Can you work these out from the model? Positions are in its coordinate system, mm. A direction names the side the tool comes from. Round coordinates to 2 decimals unless told otherwise and drop trailing zeros. Order: outer loops, then holes, each group sorted by start corner. A loop starts at its lowest first (then second) coordinate and runs counter-clockwise, first axis right, second up. Notation, with made-up numbers: (10.25, -14.75) - (59.25, -14.75) arc R32 ccw to (59.25, 16.25) - close; hole circle Ø9 at (54, 76.5). An arc over 180 degrees is marked (long way). Write item = value, one per line.
Autodesk Inventor part; units mm, degrees
ref_plane "YZ Plane" through (0, 0, 0) normal (1, 0, 0) x (0, 1, 0)
ref_plane "XZ Plane" through (0, 0, 0) normal (0, 1, 0) x (-1, 0, 0)
ref_plane "XY Plane" through (0, 0, 0) normal (0, 0, 1) x (1, 0, 0)
sketch "Sketch1" plane through (0, 0, 0) normal (0, 0, 1) x (1, 0, 0)
  circle A0 centre (0, 0) radius 107.6 construction
  arc A1 (43.4971, -89.6) -> (-43.4971, -89.6) centre (0, 0) ccw construction
  line L0 (43.4971, -89.6) -> (-43.4971, -89.6) construction
  arc A2 (-96.8589, 20.9561) -> (-43.4971, -89.0439) centre (0, 0) ccw
  line L1 (-43.4971, -89.0439) -> (0, -89.0439)
  line L2 (-96.8589, 20.9561) -> (-91.8589, 20.9561)
  arc A3 (-91.8589, 20.9561) -> (-43.4971, -83.5776) centre (0, 0) ccw
  line L3 (-43.4971, -83.5776) -> (0, -83.5776)
  line L4 (0, 99.6) -> (0, -89.6) construction
  arc A4 (43.4971, -89.0439) -> (96.8589, 20.9561) centre (0, 0) ccw
  line L5 (43.4971, -89.0439) -> (0, -89.0439)
  line L6 (96.8589, 20.9561) -> (91.8589, 20.9561)
  arc A5 (43.4971, -83.5776) -> (91.8589, 20.9561) centre (0, 0) ccw
  line L7 (43.4971, -83.5776) -> (0, -83.5776)
  dimension "d0" = 0.5
  dimension "d1" = 110
  dimension "d2" = 5
extrude "Extrusion1" add sketch "Sketch1" against normal blind 240
sketch "Sketch2" plane through (0, 0, 0) normal (0, 0, 1) x (1, 0, 0)
  line L0 (-50, -78.5776) -> (50, -78.5776) construction
  line L1 (50, -78.5776) -> (50, 21.4224) construction
  line L2 (-50, 21.4224) -> (50, 21.4224) construction
  line L3 (-50, -78.5776) -> (-50, 21.4224) construction
  arc A0 (-91.8589, 20.9561) -> (-43.4971, -83.5776) centre (0, 0) ccw
  line L4 (-51.9882, -78.5776) -> (51.9882, -78.5776)
  arc A1 (-51.9882, -78.5776) -> (-43.4971, -83.5776) centre (0, 0) ccw
  arc A2 (43.4971, -83.5776) -> (91.8589, 20.9561) centre (0, 0) ccw
  arc A3 (43.4971, -83.5776) -> (51.9882, -78.5776) centre (0, 0) ccw
  line L5 (43.4971, -83.5776) -> (-43.4971, -83.5776)
  line L6 (-43.4971, -83.5776) -> (43.4971, -83.5776)
extrude "Extrusion2" add sketch "Sketch2" against normal up to surface (240 mm away)
sketch "Sketch3" plane through (-51.9882, -78.5776, 0) normal (0, 1, 0) x (1, 0, 0)
  line L0 (0, 240) -> (103.9765, 240) construction
  line L1 (0, 0) -> (0, 240) construction
  line L2 (103.9765, 0) -> (0, 0) construction
  line L3 (103.9765, 240) -> (103.9765, 0) construction
  line L4 (94.4882, 137.5) -> (9.4882, 137.5) construction
  line L5 (9.4882, 137.5) -> (9.4882, 222.5) construction
  line L6 (9.4882, 222.5) -> (94.4882, 222.5) construction
  line L7 (94.4882, 222.5) -> (94.4882, 137.5) construction
  line L8 (1.9882, 230) -> (1.9882, 130) construction
  line L9 (1.9882, 130) -> (101.9882, 130) construction
  line L10 (101.9882, 130) -> (101.9882, 230) construction
  line L11 (101.9882, 230) -> (1.9882, 230) construction
  line L12 (94.4882, 17.5) -> (9.4882, 17.5) construction
  line L13 (9.4882, 17.5) -> (9.4882, 102.5) construction
  line L14 (9.4882, 102.5) -> (94.4882, 102.5) construction
  line L15 (94.4882, 102.5) -> (94.4882, 17.5) construction
  line L16 (1.9882, 110) -> (1.9882, 10) construction
  line L17 (1.9882, 10) -> (101.9882, 10) construction
  line L18 (101.9882, 10) -> (101.9882, 110) construction
  line L19 (101.9882, 110) -> (1.9882, 110) construction
  line L20 (11.9882, 220) -> (11.9882, 140) construction
  line L21 (11.9882, 140) -> (91.9882, 140) construction
  line L22 (91.9882, 140) -> (91.9882, 220) construction
  line L23 (91.9882, 220) -> (11.9882, 220) construction
  line L24 (11.9882, 100) -> (11.9882, 20) construction
  line L25 (11.9882, 20) -> (91.9882, 20) construction
  line L26 (91.9882, 20) -> (91.9882, 100) construction
  line L27 (91.9882, 100) -> (11.9882, 100) construction
  line L28 (-4.0118, 124) -> (107.9882, 124)
  line L29 (107.9882, 124) -> (107.9882, 236)
  line L30 (107.9882, 236) -> (-4.0118, 236)
  line L31 (-4.0118, 236) -> (-4.0118, 124)
  line L32 (-4.0118, 124) -> (107.9882, 236) construction
  line L33 (107.9882, 124) -> (-4.0118, 236) construction
  line L34 (-7.0118, 121) -> (110.9882, 121)
  line L35 (110.9882, 121) -> (110.9882, 239)
  line L36 (110.9882, 239) -> (-7.0118, 239)
  line L37 (-7.0118, 239) -> (-7.0118, 121)
  line L38 (-7.0118, 121) -> (110.9882, 239) construction
  line L39 (110.9882, 121) -> (-7.0118, 239) construction
  line L40 (-4.0118, 4) -> (107.9882, 4)
  line L41 (107.9882, 4) -> (107.9882, 116)
  line L42 (107.9882, 116) -> (-4.0118, 116)
  line L43 (-4.0118, 116) -> (-4.0118, 4)
  line L44 (-4.0118, 4) -> (107.9882, 116) construction
  line L45 (107.9882, 4) -> (-4.0118, 116) construction
  line L46 (-7.0118, 1) -> (110.9882, 1)
  line L47 (110.9882, 1) -> (110.9882, 119)
  line L48 (110.9882, 119) -> (-7.0118, 119)
  line L49 (-7.0118, 119) -> (-7.0118, 1)
  line L50 (-7.0118, 1) -> (110.9882, 119) construction
  line L51 (110.9882, 1) -> (-7.0118, 119) construction
  point P0 (51.9882, 0)
  point P1 (51.9882, 180)
  point P2 (51.9882, 60)
  dimension "d7" = 6
  dimension "d8" = 6
  dimension "d9" = 6
  dimension "d10" = 6
  dimension "d11" = 3
  dimension "d12" = 6
  dimension "d13" = 6
  dimension "d14" = 6
  dimension "d15" = 6
  dimension "d16" = 3
extrude "Extrusion3" add sketch "Sketch3" along normal blind 60
properties part number "InsertV1_3DPrint"
(1) If I drill on line 1 (Z direction, x = 25, y = -78); line 2 (X direction, y = -54.5, z = -15); line 3 (X direction, y = -64, z = -106), over which ranges is the centre line in solid material (lowest first)? Write a range as from..to.
Computed:
line_1 = -239..-236, -124..-121, -119..-116, -4..-1
line_2 = -82.77..-76.86, -59..-56, 56..59, 76.86..82.77
line_3 = -75.66..-69.15, -59..-56, 56..59, 69.15..75.66
(2) Will these pins go through, and if not, where does the flat tip stop? P1, Ø2, axis at y = -14, z = -134, coming from the -X side; P2, Ø1.1, axis at x = -21.5, z = -239.5, coming from the +Y side; P3, Ø12, axis at x = -13, y = -15, coming from the +Z side.
Computed:
P1 = -98.24
P2 = -18.58
P3 = -1
(3) If we section it at C-C (y = -2.5): Write out the boundary of the cut face in (x, z), plus the area to 3 significant figures.
Computed:
outline = (-99.07, -240) - (-94.19, -240) - (-94.19, 0) - (-99.07, 0) - close; (94.19, -240) - (99.07, -240) - (99.07, 0) - (94.19, 0) - close
area = 2,340 mm^2
(4) If we section it at A-A (y = -27): Write out the boundary of the cut face in (x, z), plus the area to 3 significant figures.
Computed:
outline = (-95.35, -240) - (-90.27, -240) - (-90.27, 0) - (-95.35, 0) - close; (-59, -239) - (59, -239) - (59, -121) - (-59, -121) - close; (-59, -119) - (59, -119) - (59, -1) - (-59, -1) - close; (90.27, -240) - (95.35, -240) - (95.35, 0) - (90.27, 0) - close; hole (-56, -236) - (56, -236) - (56, -124) - (-56, -124) - close; hole (-56, -116) - (56, -116) - (56, -4) - (-56, -4) - close
area = 5,200 mm^2
(5) If we section it at B-B (z = -156.5): Write out the boundary of the cut face in (x, y), plus the area to 3 significant figures.
Computed:
outline = (-96.86, 20.96) arc R99.1 ccw to (-43.5, -89.04) - (43.5, -89.04) arc R99.1 ccw to (96.86, 20.96) - (91.86, 20.96) arc R94.22 cw to (59, -73.46) - (59, -18.58) - (56, -18.58) - (56, -75.77) arc R94.22 cw to (51.99, -78.58) - (-51.99, -78.58) arc R94.22 cw to (-56, -75.77) - (-56, -18.58) - (-59, -18.58) - (-59, -73.46) arc R94.22 cw to (-91.86, 20.96) - close
area = 2,540 mm^2
(6) Thinking about a two-plate mould opening in Y: for faces 4 (the face through (-87.757, -34.293, -118.32)), 5 (the face through (0, -79, -240)), 6 (the face through (88.756, -44.081, -118.32)), which applies, +Y half, -Y half, draft (parallel to the pull), parting line (faces both ways), or undercut?
Computed:
face_4 = undercut
face_5 = draft
face_6 = parting line
(7) On a 3-axis mill with a long thin cutter (end or side, diameter ignored), from which of +Z, -Z, +X, -X, +Y, -Y can I reach the whole of each face in a straight line? I mean faces 1 (the face through (59, -46, -179)), 2 (the face through (-1, -49, -1)), 3 (the face through (56, -48, -59)). Say none if no direction works.
Computed:
face_1 = +Z, -Z, +Y
face_2 = +Z, +Y
face_3 = +Y
(8) If we section it at D-D (x = -30.5): Write out the boundary of the cut face in (y, z).
Computed:
outline = (-89.04, -240) - (-78.58, -240) - (-78.58, -239) - (-18.58, -239) - (-18.58, -236) - (-78.58, -236) - (-78.58, -124) - (-18.58, -124) - (-18.58, -121) - (-78.58, -121) - (-78.58, -119) - (-18.58, -119) - (-18.58, -116) - (-78.58, -116) - (-78.58, -4) - (-18.58, -4) - (-18.58, -1) - (-78.58, -1) - (-78.58, 0) - (-89.04, 0) - close
